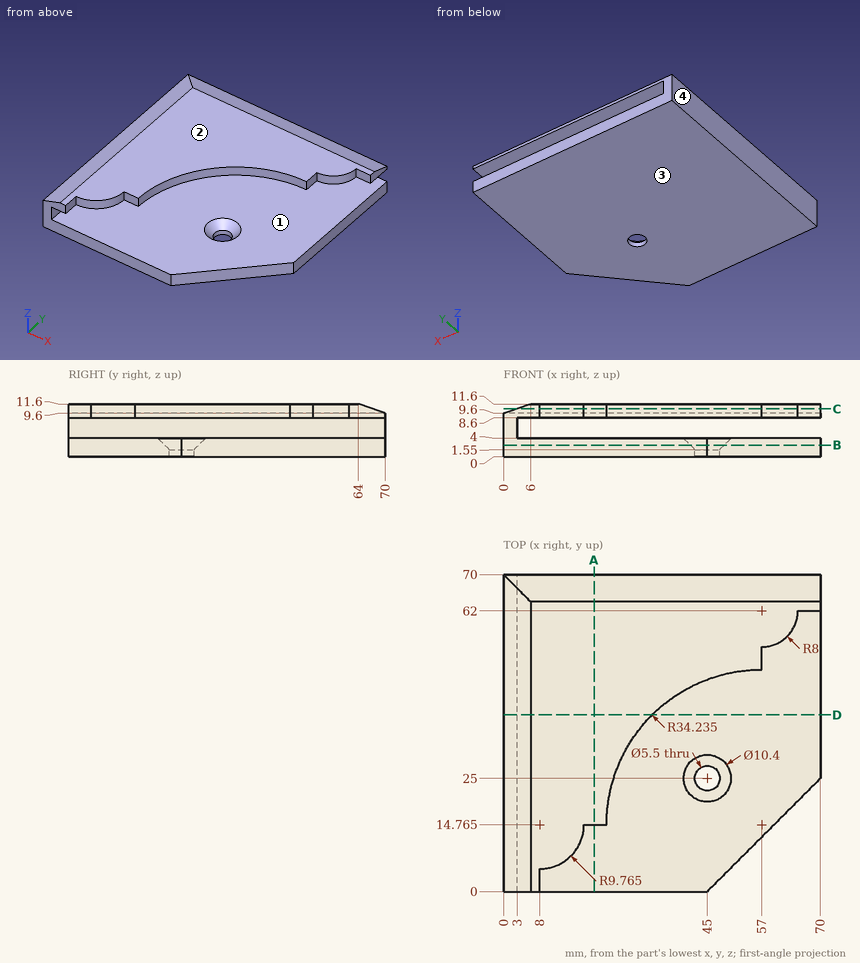
Can you work these out from the drawing? Everything is in mm from the part's minimum corner. Give positions to 0.01 mm unless a question says otherwise; leave off trailing zeros. Loops run counter-clockwise (first coordinate to the right, second up) from the corner with the lowest first, then second, coordinate; pieces in that order, holes last. Notation, with made-up numbers: (17, -8) -> (38, -8) arc R16 ccw to (38, 1) -> close; hole circle Ø6 at (15.5, -17.75). An arc over 180 degrees is marked (long way). Return JSON: item names as keys, results as strings.
Item 1: If we section it at D-D on y = 39: List the corners of the cut face in (x, z) for me.
Geometry results:
{"outline": "(0, 0) -> (70, 0) -> (70, 4) -> (3, 4) -> (3, 8.6) -> (32.82, 8.6) -> (32.82, 11.6) -> (6, 11.6) -> (0, 9.6) -> close"}
Item 2: I need wall thicknesses on L1, parallel to Z at x = 12, y = 9.5; L2, parallel to X at y = 50, z = 9.5; L3, parallel to X at y = 66.5, z = 6.5. Which ranges of each line are inside material? Lowest first, please. Write a range as from..to.
Geometry results:
{"L1": "z = 0..4, 8.6..11.6", "L2": "x = 0..57", "L3": "x = 0..3"}
Item 3: If we section it at B-B on z = 2.5: List the corners of the cut face in (x, y) for me.
Geometry results:
{"outline": "(0, 0) -> (45, 0) -> (70, 25) -> (70, 70) -> (0, 70) -> close; hole circle Ø7.4 at (45, 25)"}
Item 4: If we section it at C-C on z = 10.5: List the corners of the cut face in (x, y) for me (3 decimals), plus the area to 3 significant figures.
Geometry results:
{"outline": "(2.7, 0) -> (8, 0) -> (8, 5) arc R9.765 ccw to (17.765, 14.765) -> (22.765, 14.765) arc R34.235 cw to (57, 49) -> (57, 54) arc R8 ccw to (65, 62) -> (70, 62) -> (70, 67.3) -> (2.7, 67.3) -> close", "area": "2,200 mm²"}
Item 5: If we section it at A-A on x = 20: List the corners of the cut face in (y, z) for me (3 decimals), plus the area to 3 significant figures.
Geometry results:
{"outline": "(0, 0) -> (70, 0) -> (70, 4) -> (0, 4) -> close; (14.765, 8.6) -> (70, 8.6) -> (70, 9.6) -> (64, 11.6) -> (14.765, 11.6) -> close", "area": "440 mm²"}
Item 6: We'd pull the mould along Z, two halves only. Please class the marked faces 1, 2, 3 and 4: +Z half, -Z half, draft (parallel to the pull), parting line (faces both ways), or undercut.
Geometry results:
{"face 1": "undercut", "face 2": "+Z half", "face 3": "-Z half", "face 4": "draft"}
Item 7: I'm going to push flat-ended pins straight in: pin 1 (0.9 mm diameter, centred on x = 20, z = 10.5, fed in from -Y) (3 decimals); pin 2 (0.9 mm diameter, centred on y = 3, z = 10, fed in from +X); pin 3 (3.5 mm diameter, centred on y = 51.5, z = 10.5, fed in from +X); pin 4 (5 mm diameter, centred on x = 45, y = 25, fed in from -Z). Where does each tip first touch, or does it pass through?
Geometry results:
{"pin 1": "stops at y = 14.765", "pin 2": "stops at x = 8", "pin 3": "stops at x = 57", "pin 4": "passes through"}
